from build123d import *

# Parameters (mm, degrees)
RESSALTO_EXTRUS_O1_DEPTH   = 38
CORTE_EXTRUS_O_FINA1_START = -30.8
CORTE_EXTRUS_O_FINA1_DEPTH = 21.6
ESBO_O3_R                  = 2.25
RESSALTO_EXTRUS_O2_DEPTH   = 20
ESBO_O4_R                  = 10
RESSALTO_EXTRUS_O3_DEPTH   = 2
ESBO_O5_R                  = 1.5
CORTE_EXTRUS_O1_DEPTH      = 10


# Read off the part's stored shape, not the designer's step: Corte-Extrusão-Fina1
with BuildPart() as part:
    # Esboço1 → Ressalto-extrusão1 (new body)
    with BuildSketch(Plane.XY):
        Polygon((-21, -15.592171873), (-15.984175996, -21), (15.592171873, -21), (21, -15.984175996), (21, 15.592171873), (15.984175996, 21), (-15.592171873, 21), (-21, 15.984175996), align=None)
    extrude(amount=RESSALTO_EXTRUS_O1_DEPTH)

    # Corte-Extrusão-Fina1 outline → Corte-Extrusão-Fina1 (cut)
    with BuildSketch(Plane.XY.offset(38).offset(CORTE_EXTRUS_O_FINA1_START)):
        Polygon((15.592171873, -21), (21, -15.984175996), (21, 15.592171873), (15.984175996, 21), (-15.592171873, 21), (-21, 15.984175996), (-21, -15.592171873), (-15.984175996, -21), align=None)
        Polygon((14.605339059, 20.75), (20.75, 14.605339059), (20.75, -14.605339059), (14.605339059, -20.75), (-14.605339059, -20.75), (-20.75, -14.605339059), (-20.75, 14.605339059), (-14.605339059, 20.75), align=None, mode=Mode.SUBTRACT)
    extrude(amount=CORTE_EXTRUS_O_FINA1_DEPTH, mode=Mode.SUBTRACT)

    # Esboço3 → Ressalto-extrusão2 (add)
    with BuildSketch(Plane(origin=(0, 0, 0), x_dir=(-1, 0, 0), z_dir=(0, 0, -1))):
        with Locations(Location((0, 0, 0), (0, 0, 180))):
            Circle(ESBO_O3_R)
    extrude(amount=RESSALTO_EXTRUS_O2_DEPTH)

    # Esboço4 → Ressalto-extrusão3 (add)
    with BuildSketch(Plane(origin=(0, 0, 0), x_dir=(-1, 0, 0), z_dir=(0, 0, -1))):
        with Locations(Location((0, 0, 0), (0, 0, 180))):
            Circle(ESBO_O4_R)
    extrude(amount=RESSALTO_EXTRUS_O3_DEPTH)

    # Esboço5 → Corte-extrusão1 (cut)
    with BuildSketch(Plane(origin=(0, 0, 0), x_dir=(-1, 0, 0), z_dir=(0, 0, -1))):
        with Locations((15.5, -15.5)):
            Circle(ESBO_O5_R)
        with Locations((-15.5, -15.5)):
            Circle(ESBO_O5_R)
        with Locations((-15.5, 15.5)):
            Circle(ESBO_O5_R)
        with Locations((15.5, 15.5)):
            Circle(ESBO_O5_R)
    extrude(amount=-CORTE_EXTRUS_O1_DEPTH, mode=Mode.SUBTRACT)


solid = part.part
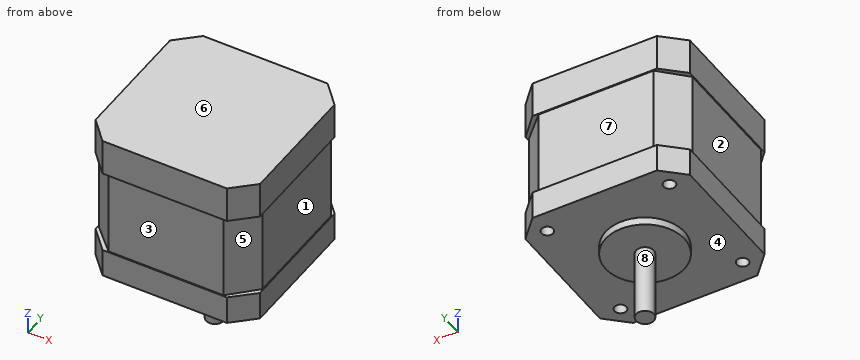
Design review of the part built by this model. Coordinates are the model's own, in mm. Face numbers are marked on the shaded views. A direction names the side the tool comes from. Coordinates: 2 decimals unless noted, no trailing zeros. Write each loop counter-clockwise with the first axis right and the second up, starting at its lowest first coordinate (ties: lowest second). Pieces come first, ordered by that corner, then holes. Notation, with made-up numbers: (64.25, -12) - (96.25, -12) arc R30 ccw to (96.25, 26) - close; hole circle Ø11 at (81.25, 71). An arc over 180 degrees is marked (long way). Use one line per item in the form item = value.
Q1. The part is to be moulded in two halves that separate along Z. For the marked faces 6, 7 and 8, say which applies: +Z half, -Z half, draft (parallel to the pull), parting line (faces both ways), or undercut.
Taken from the geometry:
face_6 = +Z half
face_7 = undercut
face_8 = draft
Q2. For probe 1 along Y at (x, z) = (-15.5, 2.75); probe 2 along Y at (x, z) = (-15, 3), list the stretches that pass through material, from the lowest coordinate up.
Taken from the geometry:
probe_1 = -21 to -17, -14 to 14, 17 to 21
probe_2 = -21 to -16.91, -14.09 to 14.09, 16.91 to 21
Q3. Consider section A-A (x = 0). Write out the cut boundary in (y, z), plus the area to 3 significant figures.
Taken from the geometry:
outline = (-21, 0) - (-10, 0) - (-10, -2) - (-2.25, -2) - (-2.25, -20) - (2.25, -20) - (2.25, -2) - (10, -2) - (10, 0) - (21, 0) - (21, 7.2) - (20.75, 7.2) - (20.75, 28.8) - (21, 28.8) - (21, 38) - (-21, 38) - (-21, 28.8) - (-20.75, 28.8) - (-20.75, 7.2) - (-21, 7.2) - close
area = 1,710 mm^2
Q4. Insertion check: pin 1 Ø8 at (x, z) = (8, 23.5) entering from +Y; pin 2 Ø2.5 at (x, y) = (15.5, -15.5) entering from -Z; pin 3 Ø17.5 at (x, z) = (0, 14) entering from +Y; pin 4 Ø3 at (x, z) = (0.5, 18.5) entering from -Y. Each pin has a flat end and moves straight along its axis. Give the tip position at first contact, or say it passes through.
Taken from the geometry:
pin_1 = 20.75
pin_2 = 10
pin_3 = 21
pin_4 = -20.75
Q5. Consider section D-D (x = -8). Write out the cut boundary in (y, z).
Taken from the geometry:
outline = (-21, 0) - (-6, 0) - (-6, -2) - (6, -2) - (6, 0) - (21, 0) - (21, 7.2) - (20.75, 7.2) - (20.75, 28.8) - (21, 28.8) - (21, 38) - (-21, 38) - (-21, 28.8) - (-20.75, 28.8) - (-20.75, 7.2) - (-21, 7.2) - close
Q6. Consider section C-C (y = -11). Write out the cut boundary in (x, z).
Taken from the geometry:
outline = (-21, 0) - (21, 0) - (21, 7.2) - (20.75, 7.2) - (20.75, 28.8) - (21, 28.8) - (21, 38) - (-21, 38) - (-21, 28.8) - (-20.75, 28.8) - (-20.75, 7.2) - (-21, 7.2) - close
Q7. Machinability: for the marked faces 1, 2, 3, 4 and 5, which of the approach directions +Z, -Z, +X, -X, +Y, -Y give a long, thin tool a straight path to every point of the face, cutting with its end or side? Answer none if there is none.
Taken from the geometry:
face_1 = +X, +Y, -Y
face_2 = -X, +Y, -Y
face_3 = +X, -X, -Y
face_4 = -Z
face_5 = +X, -Y
Q8. Consider section B-B (z = 34). Write out the cut boundary in (x, y), plus the area to 3 significant figures.
Taken from the geometry:
outline = (-21, -15.59) - (-15.98, -21) - (15.59, -21) - (21, -15.98) - (21, 15.59) - (15.98, 21) - (-15.59, 21) - (-21, 15.98) - close
area = 1,710 mm^2
